Autodesk Inventor part; units mm, degrees
ref_plane "YZ Plane" through (0, 0, 0) normal (1, 0, 0) x (0, 1, 0)
ref_plane "XZ Plane" through (0, 0, 0) normal (0, 1, 0) x (-1, 0, 0)
ref_plane "XY Plane" through (0, 0, 0) normal (0, 0, 1) x (1, 0, 0)
sketch "Sketch1" plane through (0, 0, 0) normal (1, 0, 0) x (0, 1, 0)
  line L0 (0, 0) -> (0, -7.9375)
  line L1 (0, -7.9375) -> (6.35, -7.9375)
  line L2 (6.35, -7.9375) -> (6.35, -1.5875)
  line L3 (6.35, -1.5875) -> (3.175, -4.7625)
  line L4 (3.175, -4.7625) -> (3.175, 4.7625)
  line L5 (3.175, 4.7625) -> (6.35, 1.5875)
  line L6 (6.35, 1.5875) -> (6.35, 7.9375)
  line L7 (6.35, 7.9375) -> (0, 7.9375)
  line L8 (0, 7.9375) -> (0, 0)
  dimension "d0" = 7.9375
  dimension "d1" = 7.9375
  dimension "d2" = 6.35
  dimension "d3" = 6.35
  dimension "d4" = 6.35
  dimension "d5" = 6.35
  dimension "d6" = 9.525
  dimension "d7" = 45
  dimension "d8" = 45
extrude "Extrusion1" add sketch "Sketch1" along normal blind 50.8
sketch "Sketch2" plane through (0, 0, -7.9375) normal (0, 0, -1) x (-1, 0, 0)
  point P0 (0, 0)
properties part number "Test2"
Read the model definition and answer for the solid it produces. Units are mm, in the model's axes. A direction names the side the tool comes from. Round coordinates to 2 decimals unless told otherwise and drop trailing zeros. Write each loop counter-clockwise with the first axis right and the second up, starting at its lowest first coordinate (ties: lowest second). Pieces come first, ordered by that corner, then holes.
1. The part is cut by section B-B, the plane y = 4. Determine the outline of the cut face in (x, z), then the cut area to 3 significant figures.
2. Which of the six approach directions +Z, -Z, +X, -X, +Y, -Y give full straight-line access (tool end or side, diameter ignored) to faces 1 (the face through (50.8, 3, 0)), 2 (the face through (25.04, 4.74, 3.2))?
3. Determine the mould class of faces 3 (the face through (25, 3, 7.938)), 4 (the face through (25, 6.35, -5)), 5 (the face through (25, 3.175, 0)), 6 (the face through (25, 3, -7.938)) for opening direction Z: pulls with the +Z half, pulls with the -Z half, needs draft (parallel to the pull), parting line crosses it, or undercut.
4. Given pin 1 Ø1 at (x, z) = (44.5, 3) entering from -Y, flat-ended and moving along its own axis, determine where the tip first touches the part or whether it passes through.
5. Straight lines are drawn through the part: L1, parallel to Z at x = 35.5, y = 3.25; L2, parallel to Z at x = 29.5, y = 6; L3, parallel to Y at x = 4.5, z = -1.25 (3 decimals). For each, find the intervals that lie inside material, in ascending order.
Values:
1. outline: (0, -7.94) - (50.8, -7.94) - (50.8, -3.94) - (0, -3.94) - close; (0, 3.94) - (50.8, 3.94) - (50.8, 7.94) - (0, 7.94) - close
1. area: 406 mm2
2. face 1: +Z, -Z, +X, +Y, -Y
2. face 2: +X, -X
3. face 3: pulls with the +Z half
3. face 4: needs draft
3. face 5: undercut
3. face 6: pulls with the -Z half
4. pin 1: stops at y = 0
5. L1: z = -7.94 to -4.69, 4.69 to 7.94
5. L2: z = -7.94 to -1.94, 1.94 to 7.94
5. L3: y = 0 to 3.175
